Part model, mm, in its own coordinate system. Give positions to 0.01 mm unless a question says otherwise; leave off trailing zeros. Loops run counter-clockwise (first coordinate to the right, second up) from the corner with the lowest first, then second, coordinate; pieces in that order, holes last. Notation, with made-up numbers: (-15, 49) -> (3, 49) arc R20 ccw to (3, 58) -> close; hole circle Ø6 at (62.25, 72.5). An arc over 180 degrees is marked (long way). Write item = value, one per line.
from build123d import *

# Parameters (mm, degrees)
SKETCH_1_W          = 50
SKETCH_1_H          = 148
EXTRUDE_1_DEPTH     = 25
SKETCH_2_R          = 10.5
CUT_EXTRUDE_1_DEPTH = 26
CHAMFER_1_SIZE      = 6
CHAMFER_1_SIZE2     = 10.392304845
CHAMFER_2_SIZE      = 6
CHAMFER_2_SIZE2     = 10.392304845


with BuildPart() as part:
    # Эскиз1 → Бобышка-Вытянуть1 (new body)
    with BuildSketch(Plane.XY):
        with Locations((25, 74)):
            Rectangle(SKETCH_1_W, SKETCH_1_H)
    extrude(amount=EXTRUDE_1_DEPTH)

    # Эскиз2 → Вырез-Вытянуть1 (cut, through all)
    with BuildSketch(Plane.XY.offset(25)):
        with Locations((25, 23)):
            Circle(SKETCH_2_R)
        with Locations((25, 73)):
            Circle(SKETCH_2_R)
        with Locations((25, 123)):
            Circle(SKETCH_2_R)
    extrude(amount=-CUT_EXTRUDE_1_DEPTH, mode=Mode.SUBTRACT)

    # Фаска1
    chamfer_1_edges = [part.edges().sort_by_distance(p)[0] for p in [
        (25, 0, 0),
    ]]
    chamfer_1_side = [part.faces().sort_by_distance(p)[0] for p in [
        (25, 1.562177967, 0),
    ]]
    chamfer(chamfer_1_edges, length=CHAMFER_1_SIZE, length2=CHAMFER_1_SIZE2, reference=chamfer_1_side[0])

    # Фаска2
    chamfer_2_edges = [part.edges().sort_by_distance(p)[0] for p in [
        (25, 0, 25),
    ]]
    chamfer_2_side = [part.faces().sort_by_distance(p)[0] for p in [
        (25, 1.562177967, 25),
    ]]
    chamfer(chamfer_2_edges, length=CHAMFER_2_SIZE, length2=CHAMFER_2_SIZE2, reference=chamfer_2_side[0])


solid = part.part
1) Slice it at D-D, the plane x = 5.5. List the corners of the cut face in (y, z).
Resolved:
outline = (0, 10.39) -> (6, 0) -> (148, 0) -> (148, 25) -> (6, 25) -> (0, 14.61) -> close
2) Slice it at B-B, the plane y = 123. List the corners of the cut face in (x, z), and give its area (3 significant figures).
Resolved:
outline = (0, 0) -> (14.5, 0) -> (14.5, 25) -> (0, 25) -> close; (35.5, 0) -> (50, 0) -> (50, 25) -> (35.5, 25) -> close
area = 725 mm²
3) Slice it at C-C, the plane z = 9. List the corners of the cut face in (x, y).
Resolved:
outline = (0, 0.8) -> (50, 0.8) -> (50, 148) -> (0, 148) -> close; hole circle Ø21 at (25, 23); hole circle Ø21 at (25, 73); hole circle Ø21 at (25, 123)
4) Drill centre lines: line 1 along Y through (x, z) = (25, 12.5); line 2 along Y through (x, z) = (25, 14.75); line 3 along X through (y, z) = (76.5, 8). Where is each one in solid material? Low to high. Write a range as [from, to].
Resolved:
line_1 = [0, 12.5], [33.5, 62.5], [83.5, 112.5], [133.5, 148]
line_2 = [0.08, 12.5], [33.5, 62.5], [83.5, 112.5], [133.5, 148]
line_3 = [0, 15.1], [34.9, 50]
5) Slice it at A-A, the plane x = 25. List the corners of the cut face in (y, z), and give its area (3 significant figures).
Resolved:
outline = (0, 10.39) -> (6, 0) -> (12.5, 0) -> (12.5, 25) -> (6, 25) -> (0, 14.61) -> close; (33.5, 0) -> (62.5, 0) -> (62.5, 25) -> (33.5, 25) -> close; (83.5, 0) -> (112.5, 0) -> (112.5, 25) -> (83.5, 25) -> close; (133.5, 0) -> (148, 0) -> (148, 25) -> (133.5, 25) -> close
area = 2,060 mm²
6) Pull direction Y, two halves, no side cores. Call faces 1 (the face through (0, 73, 12)), 2 (the face through (17.261, 30.096, 12.675)), 3 (the face through (25, 148, 12)), 4 (the face through (24.65, 2.958, 5.269)): pulls with the +Y half, pulls with the -Y half, needs draft (parallel to the pull), parting line crosses it, or undercut.
Resolved:
face_1 = needs draft
face_2 = undercut
face_3 = pulls with the +Y half
face_4 = pulls with the -Y half
